```python
from build123d import *

# Parameters (mm, degrees)
F0_W     = 76.2
F0_H     = 76.2
F1_DEPTH = 76.2
F2_W     = 25.4
F2_H     = 23.510535
F3_DEPTH = 12.7
F4_R     = 12.7
F5_DEPTH = 12.7


with BuildPart() as f1:
    # F0 (on Front) → F1 (new body)
    with BuildSketch(Plane.XZ):
        with Locations((23.867505, 35.862454)):
            Rectangle(F0_W, F0_H)
    extrude(amount=F1_DEPTH)

    # F2 (on face) → F3 (join)
    with BuildSketch(Plane.XZ.offset(76.2)):
        with Locations((23.867505, 34.917721)):
            Rectangle(F2_W, F2_H)
    extrude(amount=F3_DEPTH)

    # F4 (on face) → F5 (join)
    with BuildSketch(Plane.YZ.offset(61.967505)):
        with Locations((-38.1, 35.862454)):
            Circle(F4_R)
    extrude(amount=F5_DEPTH)


solid = f1.part
```
The model under review builds one solid part; all positions refer to its coordinate system, in mm. A direction names the side the tool comes from. Round coordinates to 2 decimals unless told otherwise and drop trailing zeros. Loops run counter-clockwise (first coordinate to the right, second up) from the corner with the lowest first, then second, coordinate; pieces in that order, holes last. Notation, with made-up numbers: (74.25, -5.75) -> (102.25, -5.75) arc R19 ccw to (102.25, 8.25) -> close; hole circle Ø10 at (-30.5, -10). An arc over 180 degrees is marked (long way). Answer as a JSON object with one key per item and string values. Group by question number.
1) We need section C-C on z = 18.5. Write out the cut boundary in (x, y), then the cut area to 3 significant figures.
2) For line 1 (X direction, y = -25.5, z = 65.5); line 2 (Y direction, x = -7.5, z = 19.5); line 3 (X direction, y = -80.5, z = 39), list the stretches that pass through material, from the lowest coordinate up. Write a range as [from, to].
3) For faces 1 (the face through (24, -82, 46.673)), 2 (the face through (11.168, -82, 35)), 3 (the face through (61.968, -38, 18)), list the 3-axis set-ups (+Z, -Z, +X, -X, +Y, -Y) from which the entire face can be reached by the end or side of a thin tool; tool diameter is ignored.
4) We need section B-B on x = 32.5. Write out the cut boundary in (y, z).
5) We need section D-D on y = -53. Write out the cut boundary in (x, z).
6) We need section A-A on y = -38.1. Write out the cut boundary in (x, z), then the cut area to 3 significant figures.
7) For pin 1 Ø6.5 at (x, y) = (20, -85.5) entering from -Z; pin 2 Ø4 at (x, y) = (26, -83.5) entering from +Z; pin 3 Ø8 at (y, z) = (-31.5, 63) entering from +X, all flat-tipped, find the tip position at first contact; note any pin that passes through.
Result set:
{
 "1": {"outline": "(-14.23, -76.2) -> (61.97, -76.2) -> (61.97, 0) -> (-14.23, 0) -> close", "area": "5,810 mm²"},
 "2": {"line 1": "[-14.23, 61.97]", "line 2": "[-76.2, 0]", "line 3": "[11.17, 36.57]"},
 "3": {"face 1": "+Z, +X, -X, -Y", "face 2": "+Z, -Z, -X, -Y", "face 3": "+X"},
 "4": {"outline": "(-88.9, 23.16) -> (-76.2, 23.16) -> (-76.2, -2.24) -> (0, -2.24) -> (0, 73.96) -> (-76.2, 73.96) -> (-76.2, 46.67) -> (-88.9, 46.67) -> close"},
 "5": {"outline": "(-14.23, -2.24) -> (61.97, -2.24) -> (61.97, 73.96) -> (-14.23, 73.96) -> close"},
 "6": {"outline": "(-14.23, -2.24) -> (61.97, -2.24) -> (61.97, 23.16) -> (74.67, 23.16) -> (74.67, 48.56) -> (61.97, 48.56) -> (61.97, 73.96) -> (-14.23, 73.96) -> close", "area": "6,130 mm²"},
 "7": {"pin 1": "z = 23.16", "pin 2": "z = 46.67", "pin 3": "x = 61.97"}
}
